Part model, mm, in its own coordinate system. A direction names the side the tool comes from. Round coordinates to 2 decimals unless told otherwise and drop trailing zeros. Loops run counter-clockwise (first coordinate to the right, second up) from the corner with the lowest first, then second, coordinate; pieces in that order, holes last.
from build123d import *

# Parameters (mm, degrees)
BOSS_EXTRUDE1_DEPTH    = 25.4
FILLET1_R              = 2.54
F_10_CLEARANCE_HOLE1_D = 5.1054
F_10_CLEARANCE_HOLE2_D = 5.1054


with BuildPart() as part:
    # Sketch1 → Boss-Extrude1 (new body)
    with BuildSketch(Plane.XY):
        Polygon((0, 0), (0, 50.8), (-3.175, 50.8), (-3.175, 3.175), (-57.15, 3.175), (-57.15, 0), align=None)
    extrude(amount=BOSS_EXTRUDE1_DEPTH)

    # Fillet1
    fillet1_edges = [part.edges().sort_by_distance(p)[0] for p in [
        (-1.5875, 50.8, 25.4),
        (-57.15, 1.5875, 25.4),
        (-57.15, 1.5875, 0),
        (-1.5875, 50.8, 0),
    ]]
    fillet(fillet1_edges, radius=FILLET1_R)

    # #10 Clearance Hole1 (through all)
    with Locations(Plane.ZY.offset(3.175)):
        with Locations((12.7, 38.1), (12.7, 25.4), (12.7, 12.7)):
            Hole(F_10_CLEARANCE_HOLE1_D / 2)

    # #10 Clearance Hole2 (through all)
    with Locations(Plane(origin=(0, 3.175, 0), x_dir=(1, 0, 0), z_dir=(0, 1, 0))):
        with Locations((-19.05, -12.7), (-31.75, -12.7), (-44.45, -12.7)):
            Hole(F_10_CLEARANCE_HOLE2_D / 2)


solid = part.part
1) Slice it at D-D, the plane z = 9. Give the cut face in (x, y) (3 decimals), then the cut area to 3 significant figures.
Values:
outline: (-57.15, 0) - (0, 0) - (0, 50.8) - (-3.175, 50.8) - (-3.175, 3.175) - (-57.15, 3.175) - close
area: 333 mm2
2) Wall check: line 1 along X through (y, z) = (1, 12.7); line 2 along Z through (x, y) = (-44.45, 1.4); line 3 along X through (y, z) = (31.5, 6) (3 decimals). Give the ranges that are in metal, low to high.
Values:
line 1: x = -57.15 to -47, -41.9 to -34.3, -29.2 to -21.6, -16.5 to 0
line 2: z = 0 to 10.15, 15.25 to 25.4
line 3: x = -3.175 to 0
3) Slice it at B-B, the plane z = 12.7. Give the number of separate pieces and of enclosed holes in the cut face, then the cut area to 3 significant figures.
Values:
separate pieces: 7
enclosed holes: 0
area: 235 mm2
4) Slice it at A-A, the plane y = 12.7. Give the cut face in (x, z) (3 decimals).
Values:
outline: (-3.175, 0) - (0, 0) - (0, 10.147) - (-3.175, 10.147) - close; (-3.175, 15.253) - (0, 15.253) - (0, 25.4) - (-3.175, 25.4) - close
5) Slice it at C-C, the plane x = -31.75. Give the cut face in (y, z) (3 decimals), then the cut area to 3 significant figures.
Values:
outline: (0, 0) - (3.175, 0) - (3.175, 10.147) - (0, 10.147) - close; (0, 15.253) - (3.175, 15.253) - (3.175, 25.4) - (0, 25.4) - close
area: 64.4 mm2
6) Drop flat-ended pins along their axis: pin 1 Ø4 at (y, z) = (38.1, 12.7) entering from -X; pin 2 Ø5 at (y, z) = (9, 14) entering from +X; pin 3 Ø7.5 at (y, z) = (33, 17) entering from -X (3 decimals); pin 4 Ø10 at (x, z) = (-15, 8) entering from +Y (3 decimals). Give the stop position or say it passes through.
Values:
pin 1: passes through
pin 2: stops at x = 0
pin 3: stops at x = -3.175
pin 4: stops at y = 3.175
7) Tool access for faces 5 (the face through (-3.175, 27, 15)), 6 (the face through (-34.185, 1.565, 11.933)): list every direction of +Z, -Z, +X, -X, +Y, -Y with a clear straight run to the whole face (end or side of a thin tool).
Values:
face 5: +Z, -Z, -X, +Y
face 6: +Y, -Y
8) Mould opens along Y. For faces 1 (the face through (-1.61, 50.076, 24.636)), 2 (the face through (-29, 0, 13)), 3 (the face through (0, 25, 10)), 4 (the face through (-1.565, 27.552, 11.328)) say: released by +Y, released by -Y, zero draft, split by the parting line, or undercut.
Values:
face 1: released by +Y
face 2: released by -Y
face 3: zero draft
face 4: undercut
